Could you check a few things on this model? Use its own coordinates, in mm. A direction names the side the tool comes from. Give positions to 0.01 mm unless a question says otherwise; leave off trailing zeros. Order: outer loops, then holes, each group sorted by start corner. A loop starts at its lowest first (then second) coordinate and runs counter-clockwise, first axis right, second up.
(1) Imagine slicing it at D-D, the plane y = 0.5. State how many separate pieces and enclosed holes the cut face has, then the cut area to 3 significant figures.
(2) If I drill on probe 1 along X at (y, z) = (1.15, -107) (3 decimals); probe 2 along X at (y, z) = (0.4, 17.15); probe 3 along X at (y, z) = (0.7, -4), over which ranges is the centre line in solid material (lowest first)?
(3) Imagine slicing it at B-B, the plane z = -21. Write out the boundary of the cut face in (x, y) (3 decimals), then the cut area to 3 significant figures.
(4) If we mould it in two halves opening along Z, with no side actions, what happens to faces 4 (the flat face through (39, 0, -63)), 5 (the cylindrical face through (58.668, 0.616, 5.788))? For each: released by +Z, released by -Z, zero draft, split by the parting line, or undercut.
(5) Will this pin go through, and if not, where does the flat tip stop? pin 1 (15 mm diameter, centred on x = 42.5, z = -136.5, fed in from +Y).
(6) Imagine slicing it at C-C, the plane x = 24.95. Write out the boundary of the cut face in (y, z), then the cut area to 3 significant figures.
(7) On a 3-axis mill with a long thin cutter (end or side, diameter ignored), from which of +Z, -Z, +X, -X, +Y, -Y can I reach the whole of each face in a straight line? I mean faces 1 (the cylindrical face through (43.966, 0.74, -86.646)), 2 (the flat face through (39, 1.25, -143)), 3 (the flat face through (39, 1.25, 15)). Say none if no direction works.
(8) Imagine slicing it at A-A, the plane z = 5.3. Write out the boundary of the cut face in (x, y), then the cut area to 3 significant figures.
from build123d import *

# Parameters (mm, degrees)
CROQUIS2_W                 = 80
CROQUIS2_H                 = 128
SALIENTE_EXTRUIR1_DEPTH    = 1.5
CROQUIS1_W                 = 80
CROQUIS1_H                 = 30
SALIENTE_EXTRUIR2_DEPTH    = 1.25
CROQUIS6_R                 = 3.75
CORTAR_EXTRUIR1_DEPTH      = 5.25
CORTAR_EXTRUIR2_DEPTH      = 10
CORTAR_EXTRUIR2_DEPTH_BACK = 10
CROQUIS8_R                 = 3.75
CROQUIS10_R                = 7.565
CROQUIS10_R_2              = 1.5
CROQUIS10_R_3              = 3.6
CROQUIS10_R_4              = 4
CROQUIS10_R_5              = 8.5
CORTAR_EXTRUIR4_DEPTH      = 178.105194729


with BuildPart() as part:
    # Croquis2 → Saliente-Extruir1 (new body)
    with BuildSketch(Plane(origin=(0, 0, 0), x_dir=(1, 0, 0), z_dir=(0, 1, 0))):
        with Locations((40, 64)):
            Rectangle(CROQUIS2_W, CROQUIS2_H)
    extrude(amount=SALIENTE_EXTRUIR1_DEPTH)

    # Croquis1 → Saliente-Extruir2 (add)
    with BuildSketch(Plane.XZ):
        with Locations((40, 15)):
            Rectangle(CROQUIS1_W, CROQUIS1_H)
        with Locations((40, -143)):
            Rectangle(CROQUIS1_W, CROQUIS1_H)
    extrude(amount=-SALIENTE_EXTRUIR2_DEPTH)

    # Croquis6 → Cortar-Extruir1 (cut)
    with BuildSketch(Plane.XZ):
        with Locations(Location((24.95, 5.3, 0), (0, 0, 270))):
            Circle(CROQUIS6_R)
        with Locations(Location((54.95, 5.3, 0), (0, 0, 270))):
            Circle(CROQUIS6_R)
        with Locations(Location((39.95, 5.3, 0), (0, 0, 270))):
            Circle(CROQUIS6_R)
    extrude(amount=-CORTAR_EXTRUIR1_DEPTH, mode=Mode.SUBTRACT)

    # Croquis8 → Cortar-Extruir2 (cut, two sides: drawn at the far end of the back side and taken through both)
    with BuildSketch(Plane(origin=(0, 0, 0), x_dir=(1, 0, 0), z_dir=(0, 1, 0)).offset(-CORTAR_EXTRUIR2_DEPTH_BACK)):
        with Locations(Location((24.95, 4.5, 0), (0, 0, 90))):
            Circle(CROQUIS8_R)
        with Locations(Location((39.95, 4.5, 0), (0, 0, 90))):
            Circle(CROQUIS8_R)
        with Locations(Location((54.95, 4.5, 0), (0, 0, 90))):
            Circle(CROQUIS8_R)
    extrude(amount=CORTAR_EXTRUIR2_DEPTH + CORTAR_EXTRUIR2_DEPTH_BACK, mode=Mode.SUBTRACT)

    # Croquis10 → Cortar-Extruir4 (cut, through all)
    with BuildSketch(Plane(origin=(0, 0, 0), x_dir=(1, 0, 0), z_dir=(0, 1, 0))):
        with Locations(Location((65.2, 21, 0), (0, 0, 270))):
            Circle(CROQUIS10_R)
        with Locations(Location((14.8, 21, 0), (0, 0, 90))):
            Circle(CROQUIS10_R)
        with Locations(Location((65.8, -17.15, 0), (0, 0, 270))):
            Circle(CROQUIS10_R_2)
        with Locations(Location((63.75, -23.74, 0), (0, 0, 270))):
            Circle(CROQUIS10_R_3)
        with Locations(Location((48.28, -26.35, 0), (0, 0, 270))):
            Circle(CROQUIS10_R_2)
        with Locations(Location((31.72, -26.35, 0), (0, 0, 90))):
            Circle(CROQUIS10_R_2)
        with Locations(Location((16.25, -23.74, 0), (0, 0, 90))):
            Circle(CROQUIS10_R_3)
        with Locations(Location((14.2, -17.15, 0), (0, 0, 90))):
            Circle(CROQUIS10_R_2)
        with Locations(Location((17.87, 64, 0), (0, 0, 270))):
            Circle(CROQUIS10_R_4)
        with Locations(Location((40, 86.125, 0), (0, 0, 270))):
            Circle(CROQUIS10_R_4)
        with Locations(Location((62.13, 64, 0), (0, 0, 90))):
            Circle(CROQUIS10_R_4)
        with Locations(Location((65.8, 145.15, 0), (0, 0, 90))):
            Circle(CROQUIS10_R_2)
        with Locations(Location((63.75, 151.74, 0), (0, 0, 90))):
            Circle(CROQUIS10_R_3)
        with Locations(Location((48.28, 154.35, 0), (0, 0, 90))):
            Circle(CROQUIS10_R_2)
        with Locations(Location((14.2, 145.15, 0), (0, 0, 270))):
            Circle(CROQUIS10_R_2)
        with Locations(Location((31.72, 154.35, 0), (0, 0, 270))):
            Circle(CROQUIS10_R_2)
        with Locations(Location((16.25, 151.74, 0), (0, 0, 270))):
            Circle(CROQUIS10_R_3)
        with Locations(Location((65.2, 107, 0), (0, 0, 90))):
            Circle(CROQUIS10_R)
        with Locations(Location((14.8, 107, 0), (0, 0, 270))):
            Circle(CROQUIS10_R)
        with Locations((-2, 64)):
            Circle(CROQUIS10_R_5)
    extrude(amount=CORTAR_EXTRUIR4_DEPTH, mode=Mode.SUBTRACT)


solid = part.part
Answer block:
1. separate pieces: 1
1. enclosed holes: 25
1. area: 13,600 mm2
2. probe 1: x = 0 to 7.235, 22.365 to 57.635, 72.765 to 80
2. probe 2: x = 0 to 12.7, 15.7 to 64.3, 67.3 to 80
2. probe 3: x = 0 to 21.23, 28.67 to 36.23, 43.67 to 51.23, 58.67 to 80
3. outline: (0, 0) - (7.235, 0) - (7.235, 1.5) - (0, 1.5) - close; (22.365, 0) - (57.635, 0) - (57.635, 1.5) - (22.365, 1.5) - close; (72.765, 0) - (80, 0) - (80, 1.5) - (72.765, 1.5) - close
3. area: 74.6 mm2
4. face 4: zero draft
4. face 5: undercut
5. pin 1: stops at y = 1.25
6. outline: (0, -158) - (1.25, -158) - (1.25, -128) - (1.5, -128) - (1.5, -8.25) - (0, -8.25) - close; (0, -0.75) - (1.5, -0.75) - (1.5, 0) - (1.25, 0) - (1.25, 1.55) - (0, 1.55) - close; (0, 9.05) - (1.25, 9.05) - (1.25, 30) - (0, 30) - close
6. area: 246 mm2
7. face 1: +Y, -Y
7. face 2: -Z, +X, -X, +Y
7. face 3: +Z, +X, -X, +Y
8. outline: (0, 0) - (21.2, 0) - (21.2, 1.25) - (0, 1.25) - close; (28.7, 0) - (36.2, 0) - (36.2, 1.25) - (28.7, 1.25) - close; (43.7, 0) - (51.2, 0) - (51.2, 1.25) - (43.7, 1.25) - close; (58.7, 0) - (80, 0) - (80, 1.25) - (58.7, 1.25) - close
8. area: 71.9 mm2
